from build123d import *

# Parameters (mm, degrees)
SKETCH1_W           = 78.486
SKETCH1_H           = 86.614
SKETCH1_R           = 1.5875
BOSS_EXTRUDE1_DEPTH = 2.54
SKETCH2_W           = 41.275
SKETCH2_H           = 5.08
BOSS_EXTRUDE2_DEPTH = 8.382
SKETCH4_R           = 1.27
CUT_EXTRUDE1_DEPTH  = 2.54


with BuildPart() as part:
    # Sketch1 → Boss-Extrude1 (new body)
    with BuildSketch(Plane.XY):
        with Locations((39.243, 43.307)):
            Rectangle(SKETCH1_W, SKETCH1_H)
        with Locations((6.223, 80.1116)):
            Circle(SKETCH1_R, mode=Mode.SUBTRACT)
        with Locations((72.263, 80.1116)):
            Circle(SKETCH1_R, mode=Mode.SUBTRACT)
        with Locations((72.263, 3.9116)):
            Circle(SKETCH1_R, mode=Mode.SUBTRACT)
        with Locations((6.223, 3.9116)):
            Circle(SKETCH1_R, mode=Mode.SUBTRACT)
    extrude(amount=BOSS_EXTRUDE1_DEPTH)

    # Sketch2 → Boss-Extrude2 (add)
    with BuildSketch(Plane.XY.offset(2.54)):
        with Locations((39.243, 67.564)):
            Rectangle(SKETCH2_W, SKETCH2_H)
    extrude(amount=BOSS_EXTRUDE2_DEPTH)

    # Sketch4 → Cut-Extrude1 (cut)
    with BuildSketch(Plane.XY.offset(2.54)):
        with Locations((21.082, 10.7569)):
            Circle(SKETCH4_R)
        with Locations((57.404, 7.8105)):
            Circle(SKETCH4_R)
    extrude(amount=-CUT_EXTRUDE1_DEPTH, mode=Mode.SUBTRACT)


solid = part.part
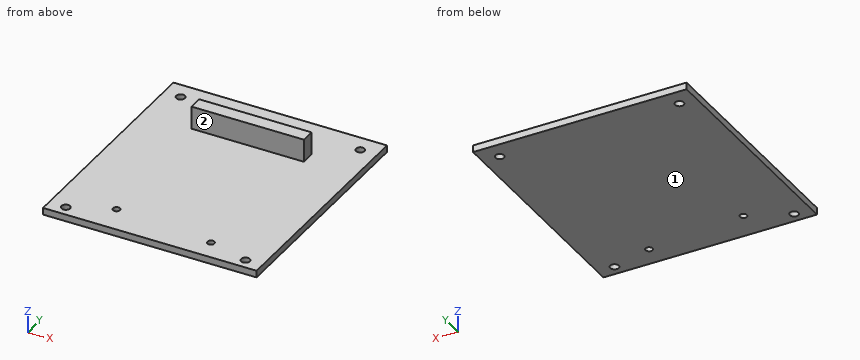
Input: part model. Units: mm. Frame: model coordinates. Face numbers are marked on the shaded views. A direction names the side the tool comes from. Give positions to 0.01 mm unless a question says otherwise; leave off trailing zeros. Write each loop counter-clockwise with the first axis right and the second up, starting at its lowest first coordinate (ties: lowest second). Pieces come first, ordered by that corner, then holes.
Q1. First-contact query: P1, Ø6.5, axis at x = 39.5, z = 6.5, coming from the -Y side; P2, Ø4, axis at y = 66.5, z = 6, coming from the +X side; P3, Ø10, axis at x = 13, y = 55.5, coming from the -Z side; P4, Ø4, axis at x = 49.5, z = 5.5, coming from the +Y side. Flat tips, straight axial feed; report the tip coordinate or a pass-through.
Q2. Set-up query: the marked faces 1 and 2. Return all of +Z, -Z, +X, -X, +Y, -Y with unobstructed straight access to the full face (end or side cutting, diameter ignored); none if empty.
Q3. Material intervals for probe 1 along Z at (x, y) = (36, 24); probe 2 along Y at (x, z) = (20, 9); probe 3 along X at (y, z) = (68.5, 3.5), sorted ascending.
Q4. Section A-A, the plane x = 39. Output: boundary loops of the cut face in (y, z).
Q5. Section C-C, the plane z = 5.5. Output: boundary loops of the cut face in (x, y).
Q6. Section B-B, the plane y = 29. Output: boundary loops of the cut face in (x, z), plus the area to 3 significant figures.
Filled in:
1. P1: stops at y = 65.02
1. P2: stops at x = 59.88
1. P3: stops at z = 0
1. P4: stops at y = 70.1
2. face 1: -Z, +X, -X, +Y, -Y
2. face 2: +Z, +X, -X, -Y
3. probe 1: z = 0 to 2.54
3. probe 2: y = 65.02 to 70.1
3. probe 3: x = 18.61 to 59.88
4. outline: (0, 0) - (86.61, 0) - (86.61, 2.54) - (70.1, 2.54) - (70.1, 10.92) - (65.02, 10.92) - (65.02, 2.54) - (0, 2.54) - close
5. outline: (18.61, 65.02) - (59.88, 65.02) - (59.88, 70.1) - (18.61, 70.1) - close
6. outline: (0, 0) - (78.49, 0) - (78.49, 2.54) - (0, 2.54) - close
6. area: 199 mm2
